from build123d import *

# Parameters (mm, degrees)
F0_R     = 13.97
F0_R_2   = 10.9982
F1_DEPTH = 12.7


with BuildPart() as f1:
    # F0 (on Top) → F1 (new body)
    with BuildSketch(Plane.XY):
        with BuildLine():
            ThreePointArc((16.1051536961, -21.2436426615), (17.3295442362, -9.9599210186), (26.5268333458, -3.3092534322))
            ThreePointArc((26.5268333458, -3.3092534322), (11.8850746566, 7.7674924981), (11.5671555945, 26.1243529429))
            ThreePointArc((11.5671555945, 26.1243529429), (2.0600739599, 20.1404593494), (-8.7790572587, 23.0908522342))
            ThreePointArc((-8.7790572587, 23.0908522342), (-12.9749986172, 7.7809801652), (-22.865745882, -4.6355904239))
            ThreePointArc((-22.865745882, -4.6355904239), (-17.4382996656, -9.7760184777), (-15.4382576825, -16.9788654894))
            ThreePointArc((-15.4382576825, -16.9788654894), (-15.7671993387, -19.9925720546), (-16.7385335967, -22.8643554087))
            ThreePointArc((-16.7385335967, -22.8643554087), (-0.5124879595, -18.0861592081), (16.1051536961, -21.2436426615))
        make_face()
        Circle(F0_R, mode=Mode.SUBTRACT)
        with BuildLine():
            ThreePointArc((-22.865745882, -4.6355904239), (-34.5827239411, -4.0025101097), (-42.649053732, -12.5244048067))
            ThreePointArc((-42.649053732, -12.5244048067), (-41.566588122, -15.7486904821), (-40.2407622083, -18.8807721477))
            ThreePointArc((-40.2407622083, -18.8807721477), (-30.3628130668, -6.022167663), (-18.4100576825, -16.9788654894))
            ThreePointArc((-18.4100576825, -16.9788654894), (-24.7565779814, -26.9449218408), (-36.4716094271, -25.4091362662))
            ThreePointArc((-36.4716094271, -25.4091362662), (-34.4220600948, -28.1233760212), (-32.1709795959, -30.672961576))
            ThreePointArc((-32.1709795959, -30.672961576), (-23.1010589715, -29.4440227054), (-16.7385335967, -22.8643554087))
            ThreePointArc((-16.7385335967, -22.8643554087), (-15.7671993387, -19.9925720546), (-15.4382576825, -16.9788654894))
            ThreePointArc((-15.4382576825, -16.9788654894), (-17.4382996656, -9.7760184777), (-22.865745882, -4.6355904239))
        make_face()
        with BuildLine():
            ThreePointArc((13.97, 33.9577309787), (13.0678918667, 38.8964658531), (10.4780741361, 43.1973663827))
            ThreePointArc((10.4780741361, 43.1973663827), (7.1445280272, 43.8720665033), (3.7691527812, 44.2899084139))
            ThreePointArc((3.7691527812, 44.2899084139), (9.011500967, 40.2627491041), (10.9982, 33.9577309787))
            ThreePointArc((10.9982, 33.9577309787), (-6.3050181253, 24.9462300117), (-3.7691527812, 44.2899084139))
            ThreePointArc((-3.7691527812, 44.2899084139), (-7.1445280272, 43.8720665033), (-10.4780741361, 43.1973663827))
            ThreePointArc((-10.4780741361, 43.1973663827), (-13.920389908, 32.7814466551), (-8.7790572587, 23.0908522342))
            ThreePointArc((-8.7790572587, 23.0908522342), (2.0600739599, 20.1404593494), (11.5671555945, 26.1243529429))
            ThreePointArc((11.5671555945, 26.1243529429), (13.3557864549, 29.8609190264), (13.97, 33.9577309787))
        make_face()
        with BuildLine():
            ThreePointArc((-40.2407622083, -18.8807721477), (-41.566588122, -15.7486904821), (-42.649053732, -12.5244048067))
            ThreePointArc((-42.649053732, -12.5244048067), (-41.5066325733, -23.9638654894), (-32.1709795959, -30.672961576))
            ThreePointArc((-32.1709795959, -30.672961576), (-34.4220600948, -28.1233760212), (-36.4716094271, -25.4091362662))
            ThreePointArc((-36.4716094271, -25.4091362662), (-38.9329782784, -22.4779654894), (-40.2407622083, -18.8807721477))
        make_face()
        with BuildLine():
            ThreePointArc((3.7691527812, 44.2899084139), (7.1445280272, 43.8720665033), (10.4780741361, 43.1973663827))
            ThreePointArc((10.4780741361, 43.1973663827), (0, 47.9277309787), (-10.4780741361, 43.1973663827))
            ThreePointArc((-10.4780741361, 43.1973663827), (-7.1445280272, 43.8720665033), (-3.7691527812, 44.2899084139))
            ThreePointArc((-3.7691527812, 44.2899084139), (0, 44.9559309787), (3.7691527812, 44.2899084139))
        make_face()
        with BuildLine():
            ThreePointArc((43.3782576825, -16.9788654894), (43.1947514501, -14.7219894197), (42.649053732, -12.5244048067))
            ThreePointArc((42.649053732, -12.5244048067), (41.566588122, -15.7486904821), (40.2407622083, -18.8807721477))
            ThreePointArc((40.2407622083, -18.8807721477), (38.9329782784, -22.4779654894), (36.4716094271, -25.4091362662))
            ThreePointArc((36.4716094271, -25.4091362662), (34.4220600948, -28.1233760212), (32.1709795959, -30.672961576))
            ThreePointArc((32.1709795959, -30.672961576), (40.2192734796, -25.8266243827), (43.3782576825, -16.9788654894))
        make_face()
        with BuildLine():
            ThreePointArc((40.2407622083, -18.8807721477), (41.566588122, -15.7486904821), (42.649053732, -12.5244048067))
            ThreePointArc((42.649053732, -12.5244048067), (36.3407102993, -4.8503041272), (26.5268333458, -3.3092534322))
            ThreePointArc((26.5268333458, -3.3092534322), (17.3295442362, -9.9599210186), (16.1051536961, -21.2436426615))
            ThreePointArc((16.1051536961, -21.2436426615), (22.3369828781, -29.0270177395), (32.1709795959, -30.672961576))
            ThreePointArc((32.1709795959, -30.672961576), (34.4220600948, -28.1233760212), (36.4716094271, -25.4091362662))
            ThreePointArc((36.4716094271, -25.4091362662), (19.4422013311, -12.3271857883), (40.4064576825, -16.9788654894))
            ThreePointArc((40.4064576825, -16.9788654894), (40.3649555088, -17.9334208737), (40.2407622083, -18.8807721477))
        make_face()
        Circle(F0_R)
        Circle(F0_R_2, mode=Mode.SUBTRACT)
    extrude(amount=F1_DEPTH)


solid = f1.part
Can you work these out from the model? Positions are in its coordinate system, mm. Round coordinates to 2 decimals unless told otherwise and drop trailing zeros. Loops run counter-clockwise (first coordinate to the right, second up) from the corner with the lowest first, then second, coordinate; pieces in that order, holes last. Notation, with made-up numbers: (-24.75, 3) - (26.25, 3) arc R13 cw to (26.25, 18) - close; hole circle Ø11 at (30.5, 70). An arc over 180 degrees is marked (long way). Write item = value, one per line. Start each with the question number.
(1) If I drill on probe 1 along Y at (x, z) = (29, 10.5); probe 2 along Y at (x, z) = (-8.5, 10.25); probe 3 along X at (y, z) = (-15, 6), over which ranges is the centre line in solid material (lowest first)? Write a range as [from, to].
(2) If we section it at B-B (x = 2): Please give me the cut outline in (y, z).
(3) If we section it at A-A (y = -1.5): Please give me the cut outline in (x, z), and give its area (3 significant figures).
(4) If we section it at C-C (z = 2): Please give me the cut outline in (x, y).
(5) For P1, Ø3, axis at y = 29.5, z = 6.5, coming from the +X side; P2, Ø1.5, axis at y = 19, z = 6.5, coming from the +X side (3 decimals); P3, Ø6, axis at y = 22, z = 1.5, coming from the +X side, each with a flat end and sliding along its axis, tell me the tip position at first contact or that it passes through.
(6) If we section it at D-D (x = 21): Please give me the cut outline in (y, z), and give its area (3 significant figures).
(7) If we mould it in two halves opening along Y, with no side actions, what happens to faces 1 (the face through (-12.874, 7.981, 6.261)), 2 (the face through (-0.8, -18.1, 6.3)), 3 (the face through (-7, -9, 0))? For each: released by +Y, released by -Y, zero draft, split by the parting line, or undercut.
Ans:
q1.probe_1 = [-30.94, -27.97], [-5.99, -3.01]
q1.probe_2 = [-19.39, -6.98], [6.98, 26.98], [40.94, 45.04]
q1.probe_3 = [-43.24, -40.23], [-18.59, 18.59], [40.23, 43.24]
q2.outline = (-18.05, 0) - (-10.81, 0) - (-10.81, 12.7) - (-18.05, 12.7) - close; (10.81, 0) - (23.14, 0) - (23.14, 12.7) - (10.81, 12.7) - close; (44.77, 0) - (47.78, 0) - (47.78, 12.7) - (44.77, 12.7) - close
q3.outline = (-19.52, 0) - (-10.9, 0) - (-10.9, 12.7) - (-19.52, 12.7) - close; (10.9, 0) - (21.22, 0) - (21.22, 12.7) - (10.9, 12.7) - close
q3.area = 241 mm²
q4.outline = (-22.87, -4.64) arc R13.97 ccw (long way) to (-16.74, -22.86) arc R36.01 cw to (16.11, -21.24) arc R13.97 ccw (long way) to (26.53, -3.31) arc R20.98 cw to (11.57, 26.12) arc R13.97 ccw (long way) to (-8.78, 23.09) arc R39.45 cw to start; hole circle Ø22 at (-29.41, -16.98); hole circle Ø22 at (0, 0); hole circle Ø22 at (0, 33.96); hole circle Ø22 at (29.41, -16.98)
q5.P1 = 13.65
q5.P2 = 9.755
q5.P3 = 11.08
q6.outline = (-28.14, 0) - (-24.07, 0) - (-24.07, 12.7) - (-28.14, 12.7) - close; (-9.89, 0) - (-1.39, 0) - (-1.39, 12.7) - (-9.89, 12.7) - close
q6.area = 160 mm²
q7.face_1 = undercut
q7.face_2 = released by -Y
q7.face_3 = zero draft
